```python
from build123d import *

# Parameters (mm, degrees)
SKETCH1_W           = 82.539998569
SKETCH1_H           = 65.04
BOSS_EXTRUDE1_DEPTH = 43.18
SHELL1_T            = 2.54
CUT_EXTRUDE2_DEPTH  = 124.028758627
SKETCH7_W           = 87.619998569
SKETCH7_H           = 43.18
BOSS_EXTRUDE2_DEPTH = 2.54
CUT_EXTRUDE3_DEPTH  = 2.54
CUT_EXTRUDE4_DEPTH  = 2.54
SKETCH10_W          = 1.27
SKETCH10_H          = 35.56
CUT_EXTRUDE5_DEPTH  = 2.54
SKETCH11_W          = 12.7
SKETCH11_H          = 2.54
BOSS_EXTRUDE3_DEPTH = 12.7
CUT_EXTRUDE7_DEPTH  = 125.717897357
SKETCH13_W          = 12.7
SKETCH13_H          = 12.7
SKETCH13_R          = 2.1
BOSS_EXTRUDE4_DEPTH = 3.175
FILLET2_R           = 3
SKETCH14_W          = 12.7
SKETCH14_H          = 12.7
SKETCH14_R          = 2.625
BOSS_EXTRUDE5_DEPTH = 7
FILLET3_R           = 2.54


with BuildPart() as part:
    # Sketch1 → Boss-Extrude1 (new body)
    with BuildSketch(Plane.XY):
        with Locations((47.599999189, 40.75)):
            Rectangle(SKETCH1_W, SKETCH1_H)
    extrude(amount=BOSS_EXTRUDE1_DEPTH)

    # Shell1
    shell1_openings = [part.faces().sort_by_distance(p)[0] for p in [
        (47.599999189, 73.27, 21.59),
        (47.599999189, 40.75, 0),
    ]]
    offset(amount=SHELL1_T, openings=shell1_openings, kind=Kind.INTERSECTION)

    # Sketch6 → Cut-Extrude2 (cut, through all)
    with BuildSketch(Plane.ZY.offset(-3.789999905)):
        Polygon((2.54, 59.03), (2.54, 73.27), (0, 73.27), (0, 59.03), (0, 3.15), (38.1, 3.15), (38.1, 19.92924), (2.54, 19.92924), align=None)
    extrude(amount=-CUT_EXTRUDE2_DEPTH, mode=Mode.SUBTRACT)

    # Sketch7 → Boss-Extrude2 (add)
    with BuildSketch(Plane(origin=(0, 73.27, 0), x_dir=(1, 0, 0), z_dir=(0, 1, 0))):
        with Locations((47.59999919, -24.13)):
            Rectangle(SKETCH7_W, SKETCH7_H)
    extrude(amount=BOSS_EXTRUDE2_DEPTH)

    # Sketch8 → Cut-Extrude3 (cut)
    with BuildSketch(Plane(origin=(0, 0, 2.54), x_dir=(-1, 0, 0), z_dir=(0, 0, -1))):
        Polygon((-65.405564728, 73.27), (-65.405564728, 74.54), (-90.139998474, 74.54), (-90.139998474, 19.92924), (-88.869998474, 19.92924), (-88.869998474, 73.27), align=None)
        Polygon((-5.059999905, 74.54), (-65.405564728, 74.54), (-65.405564728, 73.27), (-6.329999905, 73.27), (-6.329999905, 19.92924), (-5.059999905, 19.92924), align=None)
    extrude(amount=-CUT_EXTRUDE3_DEPTH, mode=Mode.SUBTRACT)

    # Sketch9 → Cut-Extrude4 (cut)
    with BuildSketch(Plane(origin=(0, 0, 38.1), x_dir=(-1, 0, 0), z_dir=(0, 0, -1))):
        Polygon((-90.139998474, 19.92924), (-90.139998474, 6.96), (-5.059999905, 6.96), (-5.059999905, 19.92924), (-6.329999905, 19.92924), (-6.329999905, 8.23), (-88.869998474, 8.23), (-88.869998474, 19.92924), align=None)
    extrude(amount=-CUT_EXTRUDE4_DEPTH, mode=Mode.SUBTRACT)

    # Sketch10 → Cut-Extrude5 (cut)
    with BuildSketch(Plane.XZ.offset(-19.92924)):
        with Locations((5.694999905, 22.86)):
            Rectangle(SKETCH10_W, SKETCH10_H)
        with Locations((89.504998474, 22.86)):
            Rectangle(SKETCH10_W, SKETCH10_H)
    extrude(amount=-CUT_EXTRUDE5_DEPTH, mode=Mode.SUBTRACT)

    # Sketch11 → Boss-Extrude3 (add)
    with BuildSketch(Plane.XZ.offset(-5.69)):
        with Locations((11.409999905, 39.37)):
            Rectangle(SKETCH11_W, SKETCH11_H)
        with Locations((83.789998474, 39.37)):
            Rectangle(SKETCH11_W, SKETCH11_H)
    extrude(amount=BOSS_EXTRUDE3_DEPTH)

    # Sketch12 → Cut-Extrude7 (cut, through all)
    with BuildSketch(Plane.XY.offset(40.64)):
        with BuildLine():
            Line((9.309999905, 0.61), (9.309999905, -1.683510845))
            ThreePointArc((9.309999905, -1.683510845), (11.409999905, -3.783510845), (13.509999905, -1.683510845))
            Line((13.509999905, -1.683510845), (13.509999905, 0.61))
            ThreePointArc((13.509999905, 0.61), (11.409999905, 2.71), (9.309999905, 0.61))
        make_face()
        with BuildLine():
            Line((81.689998474, 0.61), (81.689998474, -1.683510845))
            ThreePointArc((81.689998474, -1.683510845), (83.789998474, -3.783510845), (85.889998474, -1.683510845))
            Line((85.889998474, -1.683510845), (85.889998474, 0.61))
            ThreePointArc((85.889998474, 0.61), (83.789998474, 2.71), (81.689998474, 0.61))
        make_face()
    extrude(amount=-CUT_EXTRUDE7_DEPTH, mode=Mode.SUBTRACT)

    # Sketch13 → Boss-Extrude4 (add)
    # profile 1 of 2: a face of its own
    with BuildSketch(Plane(origin=(0, 0, 2.54), x_dir=(-1, 0, 0), z_dir=(0, 0, -1))):
        with Locations((-97.759998474, 69.46)):
            Rectangle(SKETCH13_W, SKETCH13_H)
        with Locations((-97.759998474, 69.46)):
            Circle(SKETCH13_R, mode=Mode.SUBTRACT)
    # profile 2 of 2: a face of its own
    with BuildSketch(Plane(origin=(0, 0, 2.54), x_dir=(-1, 0, 0), z_dir=(0, 0, -1))):
        with Locations((2.560000095, 69.46)):
            Rectangle(SKETCH13_W, SKETCH13_H)
        with Locations((2.560000095, 69.46)):
            Circle(SKETCH13_R, mode=Mode.SUBTRACT)
    extrude(amount=-BOSS_EXTRUDE4_DEPTH)

    # Fillet2
    fillet2_edges = [part.edges().sort_by_distance(p)[0] for p in [
        (77.439998474, 5.69, 39.37),
        (77.439998474, -7.01, 39.37),
        (90.139998474, -7.01, 39.37),
        (17.759999905, -7.01, 39.37),
        (5.059999905, -7.01, 39.37),
        (17.759999905, 5.69, 39.37),
        (3.789999905, 63.11, 4.1275),
        (-8.910000095, 63.11, 4.1275),
        (-8.910000095, 75.81, 4.1275),
        (91.409998474, 63.11, 4.1275),
        (104.109998474, 63.11, 4.1275),
        (104.109998474, 75.81, 4.1275),
        (91.409998474, 75.81, 25.7175),
        (3.789999905, 75.81, 25.7175),
        (3.789999905, 5.69, 41.91),
        (91.409998474, 5.69, 41.91),
    ]]
    fillet(fillet2_edges, radius=FILLET2_R)

    # Sketch14 → Boss-Extrude5 (add)
    # profile 1 of 4: a face of its own
    with BuildSketch(Plane.XY.offset(45.72)):
        with Locations((-2.560000095, 53.76)):
            Rectangle(SKETCH14_W, SKETCH14_H)
        with Locations((-2.560000095, 53.76)):
            Circle(SKETCH14_R, mode=Mode.SUBTRACT)
    # profile 2 of 4: a face of its own
    with BuildSketch(Plane.XY.offset(45.72)):
        with Locations((-2.560000095, 15.04)):
            Rectangle(SKETCH14_W, SKETCH14_H)
        with Locations((-2.560000095, 15.04)):
            Circle(SKETCH14_R, mode=Mode.SUBTRACT)
    # profile 3 of 4: a face of its own
    with BuildSketch(Plane.XY.offset(45.72)):
        with Locations((97.759998474, 15.04)):
            Rectangle(SKETCH14_W, SKETCH14_H)
        with Locations(Location((97.759998474, 15.04, 0), (0, 0, 180))):
            Circle(SKETCH14_R, mode=Mode.SUBTRACT)
    # profile 4 of 4: a face of its own
    with BuildSketch(Plane.XY.offset(45.72)):
        with Locations((97.759998474, 53.76)):
            Rectangle(SKETCH14_W, SKETCH14_H)
        with Locations(Location((97.759998474, 53.76, 0), (0, 0, 180))):
            Circle(SKETCH14_R, mode=Mode.SUBTRACT)
    extrude(amount=-BOSS_EXTRUDE5_DEPTH)

    # Fillet3
    fillet3_edges = [part.edges().sort_by_distance(p)[0] for p in [
        (91.409998474, 8.69, 42.22),
        (3.789999905, 60.11, 42.22),
        (3.789999905, 47.41, 42.22),
        (-8.910000095, 47.41, 42.22),
        (-8.910000095, 60.11, 42.22),
        (3.789999905, 21.39, 42.22),
        (3.789999905, 8.69, 42.22),
        (-8.910000095, 8.69, 42.22),
        (-8.910000095, 21.39, 42.22),
        (91.409998474, 21.39, 42.22),
        (104.109998474, 21.39, 42.22),
        (104.109998474, 8.69, 42.22),
        (91.409998474, 47.41, 42.22),
        (91.409998474, 60.11, 42.22),
        (104.109998474, 60.11, 42.22),
        (104.109998474, 47.41, 42.22),
    ]]
    fillet(fillet3_edges, radius=FILLET3_R)


solid = part.part
```
Can you work these out from the model? Positions are in its coordinate system, mm. A direction names the side the tool comes from. Coordinates: 2 decimals unless noted, no trailing zeros. Loops run counter-clockwise (first coordinate to the right, second up) from the corner with the lowest first, then second, coordinate; pieces in that order, holes last. Notation, with made-up numbers: M 54.5,-13.5 L 110.5,-13.5 A21 ccw 110.5,6.5 Z; hole C 19,41.25 d3. An arc over 180 degrees is marked long. Put each result on its own line as item: value. Start each with the question number.
(1) Which directions (+Z, -Z, +X, -X, +Y, -Y) give clear straight access to the entire face, cutting with the end or side of a thin tool? Please do faces 5 (the face through (47, 5.69, 42)), 6 (the face through (98, 63.11, 4)), 7 (the face through (90.14, 33.4, 4.6)).
(2) I need wall thicknesses on probe 1 along X at (y, z) = (15, 41); probe 2 along X at (y, z) = (15, 44); probe 3 along Y at (x, z) = (-2.56, 41) (3 decimals). Which ranges of each line are inside material? Lowest first, please.
(3) Will these pins go through, and if not, where does the flat tip stop? pin 1 Ø14.5 at (x, y) = (10.5, -1.5) entering from +Z; pin 2 Ø2.5 at (x, z) = (39, 40) entering from -Y; pin 3 Ø1 at (x, z) = (89, 26.5) entering from -Y; pin 4 Ø1 at (x, y) = (89.5, 23.5) entering from -Z.
(4) Imagine slicing it at B-B on x = -2.56. List the corners of the cut face in (y, z) for me (3 decimals).
(5) Imagine slicing it at D-D on z = 33.5. List the corners of the cut face in (x, y) for me.
(6) We'd pull the mould along Y, two halves only. Please class faces 1 (the face through (17.76, -1, 39)), 2 (the face through (48, 75.81, 24)), 3 (the face through (83.744, -3.783, 39.388)), 4 (the face through (81.69, -1, 39)): +Y half, -Y half, draft (parallel to the pull), parting line (faces both ways), or undercut.
(7) Imagine slicing it at C-C on y = 15.04. List the corners of the cut face in (x, z) for me (3 decimals), and give its area (3 significant figures).
(8) Imagine slicing it at A-A on y = 69.46. List the corners of the cut face in (x, z) for me (3 decimals), and give its area (3 significant figures).
Worked answers:
1. face 5: +Z, -Y
1. face 6: +Z, -Z, +X, -Y
1. face 7: -Z
2. probe 1: x = -8.91 to -5.18, 0.06 to 6.33, 88.87 to 95.14, 100.38 to 104.11
2. probe 2: x = -8.91 to -5.18, 0.06 to 95.14, 100.38 to 104.11
2. probe 3: y = 8.69 to 12.415, 17.665 to 21.39, 47.41 to 51.135, 56.385 to 60.11
3. pin 1: stops at z = 45.72
3. pin 2: stops at y = 5.69
3. pin 3: stops at y = 22.47
3. pin 4: stops at z = 5.08
4. outline: M 8.69,38.72 L 12.415,38.72 L 12.415,45.72 L 8.69,45.72 Z; M 17.665,38.72 L 21.39,38.72 L 21.39,45.72 L 17.665,45.72 Z; M 47.41,38.72 L 51.135,38.72 L 51.135,45.72 L 47.41,45.72 Z; M 56.385,38.72 L 60.11,38.72 L 60.11,45.72 L 56.385,45.72 Z; M 63.11,2.54 L 67.36,2.54 L 67.36,5.715 L 63.11,5.715 Z; M 71.56,2.54 L 75.81,2.54 L 75.81,5.715 L 71.56,5.715 Z
5. outline: M 3.79,19.93 L 5.06,19.93 L 5.06,22.47 L 6.33,22.47 L 6.33,73.27 L 88.87,73.27 L 88.87,22.47 L 90.14,22.47 L 90.14,19.93 L 91.41,19.93 L 91.41,72.81 A3 ccw 88.41,75.81 L 6.79,75.81 A3 ccw 3.79,72.81 Z
6. face 1: draft
6. face 2: +Y half
6. face 3: undercut
6. face 4: undercut
7. outline: M -8.91,38.72 L -5.185,38.72 L -5.185,45.72 L -8.91,45.72 Z; M 0.065,38.72 L 3.79,38.72 L 3.79,38.1 L 5.06,38.1 L 5.06,40.64 L 6.33,40.64 L 6.33,43.18 L 88.87,43.18 L 88.87,40.64 L 90.14,40.64 L 90.14,38.1 L 91.41,38.1 L 91.41,38.72 L 95.135,38.72 L 95.135,45.72 L 0.065,45.72 Z; M 100.385,38.72 L 104.11,38.72 L 104.11,45.72 L 100.385,45.72 Z
7. area: 346 mm2
8. outline: M -8.91,2.54 L -4.66,2.54 L -4.66,5.715 L -8.91,5.715 Z; M -0.46,2.54 L 5.06,2.54 L 5.06,5.08 L 6.33,5.08 L 6.33,43.18 L 88.87,43.18 L 88.87,5.08 L 90.14,5.08 L 90.14,2.54 L 95.66,2.54 L 95.66,5.715 L 91.41,5.715 L 91.41,45.72 L 3.79,45.72 L 3.79,5.715 L -0.46,5.715 Z; M 99.86,2.54 L 104.11,2.54 L 104.11,5.715 L 99.86,5.715 Z
8. area: 477 mm2
